Design review of the part built by this model. Coordinates are the model's own, in mm. Face numbers are marked on the shaded views. A direction names the side the tool comes from. Round coordinates to 2 decimals unless told otherwise and drop trailing zeros. Order: outer loops, then holes, each group sorted by start corner. A loop starts at its lowest first (then second) coordinate and runs counter-clockwise, first axis right, second up. Notation, with made-up numbers: (61.5, 81.25) - (74.5, 81.25) arc R26 ccw to (74.5, 112.25) - close; hole circle Ø1 at (0, 29). An arc over 180 degrees is marked (long way). Write item = value, one per line.
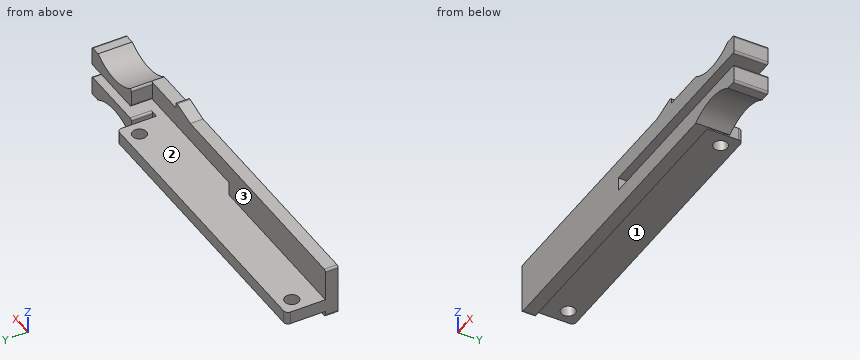
from build123d import *

# Parameters (mm, degrees)
EXTRUDE_1_DEPTH     = 3
SKETCH_4_W          = 70
SKETCH_4_H          = 3
EXTRUDE_2_DEPTH     = 9.25
CUT_EXTRUDE_1_REACH = 91.308
SKETCH_5_R          = 1.65
FILLET_1_R          = 1
EXTRUDE_3_DEPTH     = 5


with BuildPart() as part:
    # ｽｹｯﾁ2 → ﾎﾞｽ - 押し出し1 (new body)
    with BuildSketch(Plane(origin=(0, 0, 0), x_dir=(1, 0, 0), z_dir=(0, 1, 0))):
        with BuildLine():
            Line((70, 7.6), (40, 7.6))
            Line((40, 7.6), (40, 4.4))
            Line((40, 4.4), (70, 4.4))
            Line((70, 4.4), (87.5, 4.4))
            ThreePointArc((87.5, 4.4), (87.853553391, 4.253553391), (88, 3.9))
            Line((88, 3.9), (88, 0.5))
            ThreePointArc((88, 0.5), (87.853553391, 0.146446609), (87.5, 0))
            Line((87.5, 0), (85.383249581, 0))
            ThreePointArc((85.383249581, 0), (78.75, 2), (72.116750419, 0))
            Line((72.116750419, 0), (70, 0))
            Line((70, 0), (62, 0))
            Line((62, 0), (62, -0.949194177))
            ThreePointArc((62, -0.949194177), (61.80461807, -1.345688605), (61.371168675, -1.432311647))
            Line((61.371168675, -1.432311647), (56, 0))
            Line((56, 0), (0.5, 0))
            ThreePointArc((0.5, 0), (0.146446609, 0.146446609), (0, 0.5))
            Line((0, 0.5), (0, 11.5))
            ThreePointArc((0, 11.5), (0.146446609, 11.853553391), (0.5, 12))
            Line((0.5, 12), (70, 12))
            Line((70, 12), (72.116750419, 12))
            ThreePointArc((72.116750419, 12), (78.75, 10), (85.383249581, 12))
            Line((85.383249581, 12), (87.5, 12))
            ThreePointArc((87.5, 12), (87.853553391, 11.853553391), (88, 11.5))
            Line((88, 11.5), (88, 8.1))
            ThreePointArc((88, 8.1), (87.853553391, 7.746446609), (87.5, 7.6))
            Line((87.5, 7.6), (70, 7.6))
        make_face()
    extrude(amount=EXTRUDE_1_DEPTH)

    # ｽｹｯﾁ4 → ﾎﾞｽ - 押し出し2 (add)
    with BuildSketch(Plane(origin=(0, 3, 0), x_dir=(1, 0, 0), z_dir=(0, 1, 0))):
        with Locations((35, 9.1)):
            Rectangle(SKETCH_4_W, SKETCH_4_H)
    extrude(amount=EXTRUDE_2_DEPTH)

    # ｽｹｯﾁ5 → ｶｯﾄ - 押し出し1 (cut, up to next)
    with BuildSketch(Plane.XY.offset(-7.6), mode=Mode.PRIVATE) as cut_extrude_1_sk1:
        with Locations((3.45, 8.95)):
            Circle(SKETCH_5_R)
    cut_extrude_1_tool1 = extrude(cut_extrude_1_sk1.sketch, amount=-CUT_EXTRUDE_1_REACH, mode=Mode.PRIVATE) & part.part
    # ｽｹｯﾁ5 → ｶｯﾄ - 押し出し1 (cut, up to next)
    with BuildSketch(Plane.XY.offset(-7.6), mode=Mode.PRIVATE) as cut_extrude_1_sk2:
        with Locations((66.55, 8.95)):
            Circle(SKETCH_5_R)
    cut_extrude_1_tool2 = extrude(cut_extrude_1_sk2.sketch, amount=-CUT_EXTRUDE_1_REACH, mode=Mode.PRIVATE) & part.part
    add(cut_extrude_1_tool1.solids().sort_by_distance((3.45, 8.95, -7.6))[0], mode=Mode.SUBTRACT)
    add(cut_extrude_1_tool2.solids().sort_by_distance((66.55, 8.95, -7.6))[0], mode=Mode.SUBTRACT)

    # ﾌｨﾚｯﾄ1
    fillet_1_edges = [part.edges().sort_by_distance(p)[0] for p in [
        (70, 12.25, -9.1),
        (0, 12.25, -9.1),
    ]]
    fillet(fillet_1_edges, radius=FILLET_1_R)

    # ｽｹｯﾁ6 → ﾎﾞｽ - 押し出し3 (add)
    with BuildSketch(Plane(origin=(0, 3, 0), x_dir=(1, 0, 0), z_dir=(0, 1, 0))):
        with BuildLine():
            Line((88, 11.5), (88, 8.1))
            ThreePointArc((88, 8.1), (87.853553391, 7.746446609), (87.5, 7.6))
            Line((87.5, 7.6), (72.116750419, 7.6))
            ThreePointArc((72.116750419, 7.6), (71.763197029, 7.746446609), (71.616750419, 8.1))
            Line((71.616750419, 8.1), (71.616750419, 11.5))
            ThreePointArc((71.616750419, 11.5), (71.763197029, 11.853553391), (72.116750419, 12))
            ThreePointArc((72.116750419, 12), (78.75, 10), (85.383249581, 12))
            Line((85.383249581, 12), (87.5, 12))
            ThreePointArc((87.5, 12), (87.853553391, 11.853553391), (88, 11.5))
        make_face()
        with BuildLine():
            Line((88, 3.9), (88, 0.5))
            ThreePointArc((88, 0.5), (87.853553391, 0.146446609), (87.5, 0))
            Line((87.5, 0), (85.383249581, 0))
            ThreePointArc((85.383249581, 0), (78.75, 2), (72.116750419, 0))
            ThreePointArc((72.116750419, 0), (71.763197029, 0.146446609), (71.616750419, 0.5))
            Line((71.616750419, 0.5), (71.616750419, 3.9))
            ThreePointArc((71.616750419, 3.9), (71.763197029, 4.253553391), (72.116750419, 4.4))
            Line((72.116750419, 4.4), (87.5, 4.4))
            ThreePointArc((87.5, 4.4), (87.853553391, 4.253553391), (88, 3.9))
        make_face()
    extrude(amount=EXTRUDE_3_DEPTH)


solid = part.part
Item 1: Take a section at A-A, the plane x = 66.55. State the section outline as (y, z) points, and give its area (4 significant figures).
Data:
outline = (0, -12) - (3, -12) - (3, -10.6) - (7.3, -10.6) - (7.3, -7.6) - (0, -7.6) - close; (0, -4.4) - (3, -4.4) - (3, 0) - (0, 0) - close; (10.6, -10.6) - (12.25, -10.6) - (12.25, -7.6) - (10.6, -7.6) - close
area = 44.25 mm2
Item 2: For the marked faces 1, 2 and 3, list the 3-axis set-ups (+Z, -Z, +X, -X, +Y, -Y) from which the entire face can be reached by the end or side of a thin tool; tool diameter is ignored.
Data:
face_1 = -Z, -X, +Y
face_2 = +X, +Y
face_3 = +Z, -X, +Y
Item 3: Take a section at B-B, the plane x = 3.45. State the section outline as (y, z) points, and give its area (4 significant figures).
Data:
outline = (0, -12) - (3, -12) - (3, -10.6) - (7.3, -10.6) - (7.3, -7.6) - (3, -7.6) - (3, 0) - (0, 0) - close; (10.6, -10.6) - (12.25, -10.6) - (12.25, -7.6) - (10.6, -7.6) - close
area = 53.85 mm2
Item 4: Insertion check: P1, Ø3.5, axis at y = 6.5, z = -1.5, coming from the -X side; P2, Ø0.9, axis at x = 29, y = 1.5, coming from the +Z side; P3, Ø2, axis at x = 59, y = 6.5, coming from the -Z side; P4, Ø2, axis at x = 66.55, y = 8.95, coming from the +Z side. Each pin has a flat end and moves straight along its axis. Give the tip position at first contact, or say it passes through.
Data:
P1 = 71.62
P2 = 0
P3 = -10.6
P4 = through
Item 5: Take a section at D-D, the plane x = 32.5. State the section outline as (y, z) points, and give its area (4 significant figures).
Data:
outline = (0, -12) - (3, -12) - (3, -10.6) - (12.25, -10.6) - (12.25, -7.6) - (3, -7.6) - (3, 0) - (0, 0) - close
area = 63.75 mm2
Item 6: Take a section at C-C, the plane y = 5.5. State the section outline as (x, z) points, and give its area (3 significant figures).
Data:
outline = (0, -10.6) - (70, -10.6) - (70, -7.6) - (0, -7.6) - close; (71.62, -11.5) arc R0.5 ccw to (72.12, -12) arc R12 cw to (85.38, -12) - (87.5, -12) arc R0.5 ccw to (88, -11.5) - (88, -8.1) arc R0.5 ccw to (87.5, -7.6) - (72.12, -7.6) arc R0.5 ccw to (71.62, -8.1) - close; (71.62, -3.9) arc R0.5 ccw to (72.12, -4.4) - (87.5, -4.4) arc R0.5 ccw to (88, -3.9) - (88, -0.5) arc R0.5 ccw to (87.5, 0) - (85.38, 0) arc R12 cw to (72.12, 0) arc R0.5 ccw to (71.62, -0.5) - close
area = 318 mm2
Item 7: For line 1 along Z through (x, y) = (50.5, 0.75); line 2 along Y through (x, z) = (66.55, -9.5); line 3 along X through (y, z) = (9.25, -8.5), list the stretches that pass through material, from the lowest coordinate up. Write a range as [from, to].
Data:
line_1 = [-12, -7.6], [-4.4, 0]
line_2 = [0, 7.3], [10.6, 12.25]
line_3 = [0, 1.83], [5.07, 64.93], [68.17, 70]
